Input: part model. Units: mm. Frame: model coordinates. A direction names the side the tool comes from. Round coordinates to 2 decimals unless told otherwise and drop trailing zeros. Write each loop counter-clockwise with the first axis right and the second up, starting at its lowest first coordinate (ties: lowest second). Pieces come first, ordered by that corner, then holes. Notation, with made-up numbers: (-39.75, 18) -> (-18.75, 18) arc R15 ccw to (-18.75, 40) -> close; hole circle Ø11 at (-13.75, 43.25). An arc over 180 degrees is marked (long way). Write item = value, one per line. Start each with the question number.
```python
from build123d import *

# Parameters (mm, degrees)
SKETCH1_W           = 152.4
SKETCH1_H           = 152.4
BOSS_EXTRUDE1_DEPTH = 6.35
BOSS_EXTRUDE2_DEPTH = 6.35
SKETCH3_R           = 3.175
CUT_EXTRUDE1_DEPTH  = 2.54
SKETCH4_W           = 37.084
SKETCH4_H           = 72.644
CUT_EXTRUDE2_DEPTH  = 2.54
FILLET1_R           = 2.54
FILLET2_R           = 2.54
FILLET3_R           = 2.54
FILLET4_R           = 2.54


with BuildPart() as part:
    # Sketch1 → Boss-Extrude1 (new body)
    with BuildSketch(Plane(origin=(0, 0, 0), x_dir=(1, 0, 0), z_dir=(0, 1, 0))):
        with Locations((1.284269663, 24.829213483)):
            Rectangle(SKETCH1_W, SKETCH1_H)
    extrude(amount=BOSS_EXTRUDE1_DEPTH)

    # Sketch2 → Boss-Extrude2 (add)
    with BuildSketch(Plane(origin=(0, 0, 0), x_dir=(-1, 0, 0), z_dir=(0, -1, 0))):
        with BuildLine():
            ThreePointArc((-71.134269663, 97.854213483), (-74.309269663, 94.679213483), (-71.134269663, 91.504213483))
            Line((-71.134269663, 91.504213483), (-71.134269663, 97.854213483))
        make_face()
        with BuildLine():
            Line((-71.134269663, 97.854213483), (-71.134269663, 91.504213483))
            ThreePointArc((-71.134269663, 91.504213483), (-68.889205633, 92.434149453), (-67.959269663, 94.679213483))
            ThreePointArc((-67.959269663, 94.679213483), (-68.889205633, 96.924277513), (-71.134269663, 97.854213483))
        make_face()
        with BuildLine():
            ThreePointArc((68.565730337, 97.854213483), (65.390730337, 94.679213483), (68.565730337, 91.504213483))
            Line((68.565730337, 91.504213483), (68.565730337, 97.854213483))
        make_face()
        with BuildLine():
            Line((68.565730337, 97.854213483), (68.565730337, 91.504213483))
            ThreePointArc((68.565730337, 91.504213483), (70.810794367, 92.434149453), (71.740730337, 94.679213483))
            ThreePointArc((71.740730337, 94.679213483), (70.810794367, 96.924277513), (68.565730337, 97.854213483))
        make_face()
        with BuildLine():
            ThreePointArc((68.565730337, -41.845786517), (65.390730337, -45.020786517), (68.565730337, -48.195786517))
            Line((68.565730337, -48.195786517), (68.565730337, -41.845786517))
        make_face()
        with BuildLine():
            Line((68.565730337, -41.845786517), (68.565730337, -48.195786517))
            ThreePointArc((68.565730337, -48.195786517), (70.810794367, -47.265850547), (71.740730337, -45.020786517))
            ThreePointArc((71.740730337, -45.020786517), (70.810794367, -42.775722487), (68.565730337, -41.845786517))
        make_face()
        with BuildLine():
            ThreePointArc((-71.134269663, -41.845786517), (-74.309269663, -45.020786517), (-71.134269663, -48.195786517))
            Line((-71.134269663, -48.195786517), (-71.134269663, -41.845786517))
        make_face()
        with BuildLine():
            Line((-71.134269663, -41.845786517), (-71.134269663, -48.195786517))
            ThreePointArc((-71.134269663, -48.195786517), (-68.889205633, -47.265850547), (-67.959269663, -45.020786517))
            ThreePointArc((-67.959269663, -45.020786517), (-68.889205633, -42.775722487), (-71.134269663, -41.845786517))
        make_face()
    extrude(amount=BOSS_EXTRUDE2_DEPTH)

    # Sketch3 → Cut-Extrude1 (cut)
    with BuildSketch(Plane(origin=(0, 6.35, 0), x_dir=(1, 0, 0), z_dir=(0, 1, 0))):
        with Locations(Location((-68.565730337, 94.679213483, 0), (0, 0, 90))):
            Circle(SKETCH3_R)
        with Locations(Location((71.134269663, 94.679213483, 0), (0, 0, 90))):
            Circle(SKETCH3_R)
        with Locations(Location((-68.565730337, -45.020786517, 0), (0, 0, 90))):
            Circle(SKETCH3_R)
        with Locations(Location((71.134269663, -45.020786517, 0), (0, 0, 90))):
            Circle(SKETCH3_R)
    extrude(amount=-CUT_EXTRUDE1_DEPTH, mode=Mode.SUBTRACT)

    # Sketch4 → Cut-Extrude2 (cut)
    with BuildSketch(Plane(origin=(0, 6.35, 0), x_dir=(1, 0, 0), z_dir=(0, 1, 0))):
        with Locations((1.284269663, 24.829213483)):
            Rectangle(SKETCH4_W, SKETCH4_H)
    extrude(amount=-CUT_EXTRUDE2_DEPTH, mode=Mode.SUBTRACT)

    # Fillet1
    fillet1_edges = [part.edges().sort_by_distance(p)[0] for p in [
        (-17.257730337, 5.08, -61.151213483),
    ]]
    fillet(fillet1_edges, radius=FILLET1_R)

    # Fillet2
    fillet2_edges = [part.edges().sort_by_distance(p)[0] for p in [
        (19.826269663, 5.08, -61.151213483),
    ]]
    fillet(fillet2_edges, radius=FILLET2_R)

    # Fillet3
    fillet3_edges = [part.edges().sort_by_distance(p)[0] for p in [
        (-17.257730337, 5.08, 11.492786517),
    ]]
    fillet(fillet3_edges, radius=FILLET3_R)

    # Fillet4
    fillet4_edges = [part.edges().sort_by_distance(p)[0] for p in [
        (19.826269663, 5.08, 11.492786517),
    ]]
    fillet(fillet4_edges, radius=FILLET4_R)


solid = part.part
```
1. Reachability of faces 5 (the flat face through (-69, -6.35, -95)), 6 (the cylindrical face through (74.234, 5.098, 45.709)) from +Z, -Z, +X, -X, +Y, -Y: full face, straight path, thin tool, end or side. Return the list, or none.
2. Line query: line 1 along X through (y, z) = (4.25, 1); line 2 along Y through (x, z) = (57.5, -92.5); line 3 along X through (y, z) = (-3, 44.5). Output: solid intervals per line, ascending.
3. Mould query, pull axis X, two halves, no side actions, for faces 1 (the flat face through (-74.916, 3, -24)), 2 (the flat face through (77.484, 3, -24)), 3 (the flat face through (71, -6.35, 45)), 4 (the flat face through (1, 3.81, -25)). Classes: pulls with the +X half, pulls with the -X half, needs draft (parallel to the pull), parting line crosses it, or undercut.
4. Section B-B (x = 13.5). Output: boundary loops of the cut face in (y, z), then the cut area to 3 significant figures.
5. Pin query (flat end, axial travel): P1, Ø2, axis at x = 49.5, z = 3, coming from the -Y side; P2, Ø5, axis at x = 71.13, z = 45.02, coming from the +Y side. Return the tip coordinate at first contact, or that it passes through.
6. Section C-C (z = 32). Output: boundary loops of the cut face in (x, y).
7. Section A-A (y = -4.25). Output: boundary loops of the cut face in (x, z) (3 decimals).
Check sheet entries:
q1.face_5 = +Z, -Z, +X, -X, -Y
q1.face_6 = +Y
q2.line_1 = -74.92 to -17.26, 19.83 to 77.48
q2.line_2 = 0 to 6.35
q2.line_3 = -71.7 to -65.43, 68 to 74.27
q3.face_1 = pulls with the -X half
q3.face_2 = pulls with the +X half
q3.face_3 = needs draft
q3.face_4 = undercut
q4.outline = (0, -101.03) -> (6.35, -101.03) -> (6.35, -61.15) -> (3.81, -61.15) -> (3.81, 11.49) -> (6.35, 11.49) -> (6.35, 51.37) -> (0, 51.37) -> close
q4.area = 783 mm2
q5.P1 = 0
q5.P2 = 3.81
q6.outline = (-74.92, 0) -> (77.48, 0) -> (77.48, 6.35) -> (-74.92, 6.35) -> close
q7.outline = circle Ø6.35 at (-68.566, -94.679); circle Ø6.35 at (-68.566, 45.021); circle Ø6.35 at (71.134, -94.679); circle Ø6.35 at (71.134, 45.021)
